Input: part model. Units: mm. Frame: model coordinates. A direction names the side the tool comes from. Coordinates: 2 decimals unless noted, no trailing zeros. Order: outer loops, then holes, each group sorted by start corner. A loop starts at its lowest first (then second) coordinate and runs counter-clockwise, first axis right, second up. Notation, with made-up numbers: (-33.75, -7) -> (4.25, -7) arc R16 cw to (4.25, 6) -> close; hole circle Ø11 at (-6, -4). An arc over 180 degrees is marked (long way). Use one line per item in the form item = value. Start each with the question number.
1) Section query C-C on x = 42. Output: boundary loops of the cut face in (y, z), then the cut area to 3 significant figures.
2) Pin query (flat end, axial travel): pin 1 (10 mm diameter, centred on x = 36, y = 39, fed in from -Z); pin 2 (3 mm diameter, centred on x = 29.5, z = -6.5, fed in from -Y); pin 3 (5 mm diameter, centred on y = -37, z = -21.5, fed in from -X). Return the tip coordinate at first contact, or that it passes through.
3) Draft query along X for faces 1 (the cylindrical face through (3.42, 6.41, -9.39)), 2 (the flat face through (7.75, -34, 2)), 3 (the flat face through (53, -34, -11.739)). Return one class per face: pulls with the +X half, pulls with the -X half, needs draft (parallel to the pull), parting line crosses it, or undercut.
4) Access query for faces 4 (the flat face through (24, 52.5, -2)), 5 (the flat face through (16.248, -34, 2)), 6 (the cylindrical face through (26.578, 7.93, -8.975)), 7 (the flat face through (50, -46, -18)). Directions: +Z, -Z, +X, -X, +Y, -Y. A direction counts if a zero-diameter tool reaches every point of the face in a straight line with its end or side. Return the directions, or none.
5) Section query D-D on y = -62. Output: boundary loops of the cut face in (x, z).
6) Section query A-A on y = -6. Output: boundary loops of the cut face in (x, z).
7) Ray query, line 1 along X through (y, z) = (-62, 2.95); line 2 along Y through (x, z) = (6.5, -6); line 3 along Y through (x, z) = (20.5, -2). Return the intervals inside material, ascending.
8) Section query B-B on x = 52. Output: boundary loops of the cut face in (y, z), then the cut area to 3 significant figures.
from build123d import *

# Parameters (mm, degrees)
PAD_DEPTH       = 24
SKETCH_R        = 4.625
SKETCH_R_2      = 3
SKETCH_W        = 8.497862
SKETCH_H        = 16.9564
POCKET_DEPTH    = 4
SKETCH003_R     = 2.6
POCKET001_DEPTH = 13
SKETCH005_R     = 3.3
PAD001_DEPTH    = 8
SKETCH004_R     = 3.2
POCKET002_DEPTH = 3
POCKET003_DEPTH = 6
FILLET_R        = 12


with BuildPart() as part:
    # Sketch002 → Pad (new body, symmetric)
    with BuildSketch(Plane.YZ.offset(24)):
        Polygon((0, 4), (56.5, 4), (56.5, -8), (48.5, -8), (48.5, -4), (52.5, -4), (52.5, 0), (13, 0), (13, -13), (0, -13), (0, 0), (-68, 0), (-68, 4), align=None)
    extrude(amount=PAD_DEPTH, both=True)

    # Sketch (on Face13 of Pad) → Pocket (cut)
    with BuildSketch(Plane(origin=(24, -34, 4), x_dir=(-1, 0, 0), z_dir=(0, 0, 1))):
        with Locations((-12.025, 28)):
            Circle(SKETCH_R)
        with Locations((12.025, 28)):
            Circle(SKETCH_R)
        with Locations((12.025, -28)):
            Circle(SKETCH_R)
        with Locations((-12.025, -28)):
            Circle(SKETCH_R)
        with Locations((-12.024955, 15.059916)):
            Circle(SKETCH_R_2)
        with Locations((12.024955, 15.059916)):
            Circle(SKETCH_R_2)
        with Locations((12.024955, -15.059916)):
            Circle(SKETCH_R_2)
        with Locations((-12.024955, -15.059916)):
            Circle(SKETCH_R_2)
        with Locations((-12.001069, 0.0218)):
            Rectangle(SKETCH_W, SKETCH_H)
        with Locations((12.001069, -0.0218)):
            Rectangle(SKETCH_W, SKETCH_H)
    extrude(amount=-POCKET_DEPTH, mode=Mode.SUBTRACT)

    # Sketch003 (on Face30 of Pocket) → Pocket001 (cut)
    with BuildSketch(Plane(origin=(24, 0, 0), x_dir=(0, 0, -1), z_dir=(0, -1, 0))):
        with Locations((9.313336, 0)):
            Circle(SKETCH003_R)
    extrude(amount=-POCKET001_DEPTH, mode=Mode.SUBTRACT)

    # Sketch005 → Pad001 (join)
    with BuildSketch(Plane.YZ.offset(48)):
        Polygon((0, 4), (-68, 4), (-68, -26), (0, -26), (13, -26), (13, 4), align=None)
        with Locations((-49, -20)):
            Circle(SKETCH005_R, mode=Mode.SUBTRACT)
        with Locations((-19, -20)):
            Circle(SKETCH005_R, mode=Mode.SUBTRACT)
        with Locations((-34, -6.37)):
            Circle(SKETCH005_R, mode=Mode.SUBTRACT)
    extrude(amount=PAD001_DEPTH)

    # Sketch004 → Pocket002 (cut)
    with BuildSketch(Plane(origin=(24, 0, 0), x_dir=(0, 0, -1), z_dir=(0, -1, 0))):
        with Locations((9.313336, 0)):
            Circle(SKETCH004_R)
    extrude(amount=-POCKET002_DEPTH, mode=Mode.SUBTRACT)

    # Sketch006 (on Face35 of Pocket002) → Pocket003 (cut)
    with BuildSketch(Plane.YZ.offset(56)):
        Polygon((-42.8, -20), (-45.9, -14.630642), (-52.1, -14.630642), (-55.2, -20), (-52.1, -25.369358), (-45.9, -25.369358), align=None)
        Polygon((-27.8, -6.37), (-30.9, -1.000642), (-37.1, -1.000642), (-40.2, -6.37), (-37.1, -11.739358), (-30.9, -11.739358), align=None)
        Polygon((-12.8, -20), (-15.9, -14.630642), (-22.1, -14.630642), (-25.2, -20), (-22.1, -25.369358), (-15.9, -25.369358), align=None)
    extrude(amount=-POCKET003_DEPTH, mode=Mode.SUBTRACT)

    # Fillet
    fillet_edges = [part.edges().sort_by_distance(p)[0] for p in [
        (52, -68, -26),
        (52, 13, -26),
        (0, 6.5, -13),
    ]]
    fillet(fillet_edges, radius=FILLET_R)


solid = part.part
Answers below:
q1.outline = (-68, 0) -> (0, 0) -> (0, -13) -> (13, -13) -> (13, 0) -> (52.5, 0) -> (52.5, -4) -> (48.5, -4) -> (48.5, -8) -> (56.5, -8) -> (56.5, 4) -> (-68, 4) -> close
q1.area = 715 mm^2
q2.pin_1 = 0
q2.pin_2 = 0
q2.pin_3 = 48
q3.face_1 = pulls with the -X half
q3.face_2 = undercut
q3.face_3 = needs draft
q4.face_4 = +X, -X
q4.face_5 = +Z, -Z
q4.face_6 = -Y
q4.face_7 = +X
q5.outline = (0, 0) -> (7.35, 0) -> (7.35, 4) -> (0, 4) -> close; (16.6, 0) -> (31.4, 0) -> (31.4, 4) -> (16.6, 4) -> close; (40.65, 0) -> (48, 0) -> (48, -24.39) -> (56, -24.39) -> (56, 4) -> (40.65, 4) -> close
q6.outline = (0, 0) -> (7.35, 0) -> (7.35, 4) -> (0, 4) -> close; (16.6, 0) -> (31.4, 0) -> (31.4, 4) -> (16.6, 4) -> close; (40.65, 0) -> (48, 0) -> (48, -26) -> (56, -26) -> (56, 4) -> (40.65, 4) -> close
q7.line_1 = 0 to 7.35, 16.6 to 31.4, 40.65 to 56
q7.line_2 = 0 to 13, 48.5 to 56.5
q7.line_3 = 0 to 13, 52.5 to 56.5
q8.outline = (-68, -14) arc R12 ccw to (-56, -26) -> (1, -26) arc R12 ccw to (13, -14) -> (13, 4) -> (-68, 4) -> close; hole (-55.2, -20) -> (-52.1, -25.37) -> (-45.9, -25.37) -> (-42.8, -20) -> (-45.9, -14.63) -> (-52.1, -14.63) -> close; hole (-40.2, -6.37) -> (-37.1, -11.74) -> (-30.9, -11.74) -> (-27.8, -6.37) -> (-30.9, -1) -> (-37.1, -1) -> close; hole (-25.2, -20) -> (-22.1, -25.37) -> (-15.9, -25.37) -> (-12.8, -20) -> (-15.9, -14.63) -> (-22.1, -14.63) -> close
q8.area = 2,070 mm^2
